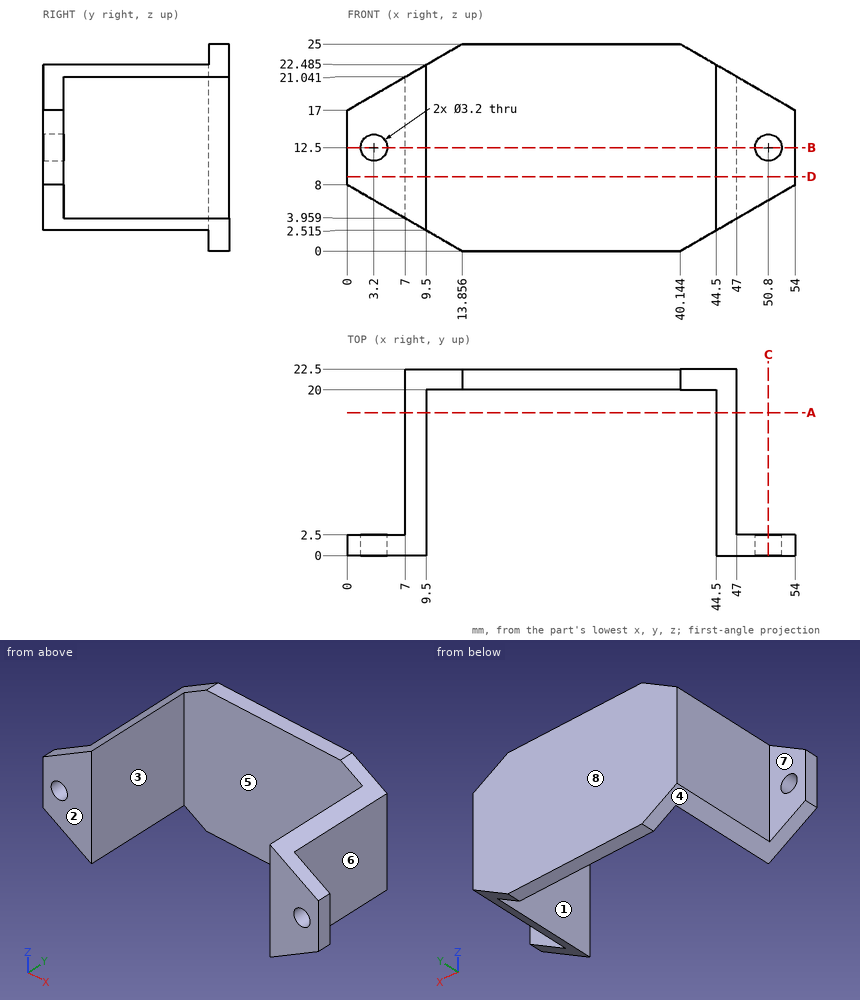
Verification items for this drawing (mm, ordinates from the low corner). A direction names the side the tool comes from. Give positions to 0.01 mm unless a question says otherwise; leave off trailing zeros. Loops run counter-clockwise (first coordinate to the right, second up) from the corner with the lowest first, then second, coordinate; pieces in that order, holes last.
(1) Depth check by flat-ended pin: pin 1 Ø3.5 at (x, z) = (3.2, 12.5) entering from +Y; pin 2 Ø5 at (y, z) = (9.5, 20) entering from -X; pin 3 Ø7.5 at (x, z) = (30.5, 11) entering from -Y. Enter the tip coordinate at first touch or a pass-through.
From the geometry:
pin 1: stops at y = 2.5
pin 2: stops at x = 7
pin 3: stops at y = 20
(2) Thickness scan on L1, parallel to X at y = 1.05, z = 12.5; L2, parallel to X at y = 17.5, z = 14; L3, parallel to Y at x = 41.5, z = 20.25. Record the ranges inside material, lowest first.
From the geometry:
L1: x = 0 to 1.6, 4.8 to 9.5, 44.5 to 49.2, 52.4 to 54
L2: x = 7 to 9.5, 44.5 to 47
L3: y = 20 to 22.5
(3) Section check B-B on z = 12.5. Record the cut outline in (x, y).
From the geometry:
outline: (0, 0) - (1.6, 0) - (1.6, 2.5) - (0, 2.5) - close; (4.8, 0) - (9.5, 0) - (9.5, 20) - (44.5, 20) - (44.5, 0) - (49.2, 0) - (49.2, 2.5) - (47, 2.5) - (47, 22.5) - (7, 22.5) - (7, 2.5) - (4.8, 2.5) - close; (52.4, 0) - (54, 0) - (54, 2.5) - (52.4, 2.5) - close
(4) Release check for a two-part mould opening along X. For the marked faces 1, 2, 3 and 4 record: released by +X, released by -X, zero draft, split by the parting line, or undercut.
From the geometry:
face 1: undercut
face 2: zero draft
face 3: undercut
face 4: released by -X
(5) Set-up check for the marked faces 5, 6, 7 and 8: record each of +Z, -Z, +X, -X, +Y, -Y from which the full face is reachable in a straight line by a thin tool's end or side.
From the geometry:
face 5: +Z, -Z, -Y
face 6: +Z, -Z, +X, +Y
face 7: +Z, -Z, -X, +Y
face 8: +Z, -Z, +X, -X, +Y
(6) Section check A-A on y = 17.25. Record the cut outline in (x, z) (1 decimal).
From the geometry:
outline: (7, 4) - (9.5, 2.5) - (9.5, 22.5) - (7, 21) - close; (44.5, 2.5) - (47, 4) - (47, 21) - (44.5, 22.5) - close
(7) Section check D-D on z = 9. Record the cut outline in (x, y).
From the geometry:
outline: (0, 0) - (9.5, 0) - (9.5, 20) - (44.5, 20) - (44.5, 0) - (54, 0) - (54, 2.5) - (47, 2.5) - (47, 22.5) - (7, 22.5) - (7, 2.5) - (0, 2.5) - close
(8) Section check C-C on x = 50.8. Record the cut outline in (y, z).
From the geometry:
outline: (0, 6.15) - (2.5, 6.15) - (2.5, 10.9) - (0, 10.9) - close; (0, 14.1) - (2.5, 14.1) - (2.5, 18.85) - (0, 18.85) - close
